from build123d import *

# Parameters (mm, degrees)
BOSS_EXTRUDE1_DEPTH = 3
SKETCH3_R           = 1.55
CUT_EXTRUDE2_DEPTH  = 3
SKETCH4_R           = 1.55
CUT_EXTRUDE4_DEPTH  = 3
SKETCH5_R           = 1.55
CUT_EXTRUDE6_DEPTH  = 3
CUT_EXTRUDE7_DEPTH  = 3


with BuildPart() as part:
    # Sketch1 → Boss-Extrude1 (new body)
    with BuildSketch(Plane.XY):
        with BuildLine():
            Line((-58.058617241, 24.191090517), (41.941382759, 24.191090517))
            ThreePointArc((41.941382759, 24.191090517), (51.941382759, 14.191090517), (41.941382759, 4.191090517))
            Line((41.941382759, 4.191090517), (-58.058617241, 4.191090517))
            ThreePointArc((-58.058617241, 4.191090517), (-68.058617241, 14.191090517), (-58.058617241, 24.191090517))
        make_face()
    extrude(amount=BOSS_EXTRUDE1_DEPTH)

    # Sketch3 → Cut-Extrude2 (cut)
    with BuildSketch(Plane.XY.offset(3)):
        with Locations((-58.058617241, 14.191090517)):
            Circle(SKETCH3_R)
    extrude(amount=-CUT_EXTRUDE2_DEPTH, mode=Mode.SUBTRACT)

    # Sketch4 → Cut-Extrude4 (cut)
    with BuildSketch(Plane(origin=(9.979459273, 1.433252018, 3), x_dir=(1, 0, 0), z_dir=(0, 0, 1))):
        with Locations((-4.038076514, 12.757838499)):
            Circle(SKETCH4_R)
    extrude(amount=-CUT_EXTRUDE4_DEPTH, mode=Mode.SUBTRACT)

    # Sketch5 → Cut-Extrude6 (cut)
    with BuildSketch(Plane(origin=(-9.979459273, 1.433252018, 0), x_dir=(-1, 0, 0), z_dir=(0, 0, -1))):
        with Locations((12.079157968, 12.757838499)):
            Circle(SKETCH5_R)
    extrude(amount=-CUT_EXTRUDE6_DEPTH, mode=Mode.SUBTRACT)

    # Sketch6 → Cut-Extrude7 (cut)
    with BuildSketch(Plane.XY.offset(3)):
        with BuildLine():
            Line((12.606210345, 17.775453704), (41.354831035, 20.463726093))
            ThreePointArc((41.354831035, 20.463726093), (48.241382759, 14.191090517), (41.354831035, 7.918454941))
            Line((41.354831035, 7.918454941), (12.606210345, 10.60672733))
            ThreePointArc((12.606210345, 10.60672733), (9.341382759, 14.191090517), (12.606210345, 17.775453704))
        make_face()
    extrude(amount=-CUT_EXTRUDE7_DEPTH, mode=Mode.SUBTRACT)


solid = part.part
Geometry: final body of the model. Coordinates: model frame, mm. A direction names the side the tool comes from. Give positions to 0.01 mm unless a question says otherwise; leave off trailing zeros. Loops run counter-clockwise (first coordinate to the right, second up) from the corner with the lowest first, then second, coordinate; pieces in that order, holes last. Notation, with made-up numbers: (72.25, 27.5) -> (96.25, 27.5) arc R22 ccw to (96.25, 38.5) -> close; hole circle Ø9 at (29.5, 13.25). An arc over 180 degrees is marked (long way). Put each result on its own line as item: value.
1. Pin query (flat end, axial travel): P1, Ø8, axis at x = -55.5, y = 21.5, coming from the -Z side; P2, Ø11.5, axis at x = 41.94, y = 14.19, coming from the +Z side. Return the tip coordinate at first contact, or that it passes through.
Taken from the geometry:
P1: stops at z = 0
P2: passes through
2. Cut plane B-B (y = 5.5). Return the cut outline in (x, z), plus the area to 3 significant figures.
Taken from the geometry:
outline: (-63, 0) -> (46.89, 0) -> (46.89, 3) -> (-63, 3) -> close
area: 330 mm2
3. Ray query, line 1 along Y through (x, z) = (42.5, 0.55); line 2 along X through (y, z) = (16.25, 1.05); line 3 along X through (y, z) = (14.75, 2.85). Return the intervals inside material, ascending. Write a range as [from, to].
Taken from the geometry:
line 1: y = [4.21, 7.92], [20.47, 24.18]
line 2: x = [-67.84, 9.99], [47.9, 51.73]
line 3: x = [-68.04, -59.5], [-56.61, -23.5], [-20.61, 4.5], [7.39, 9.39], [48.22, 51.93]
4. Pull-direction query (Y, two-part tool) for faces 1 (the flat face through (-7, 4.191, 1)), 2 (the cylindrical face through (48.24, 14.34, 1.52)), 3 (the cylindrical face through (-68.056, 13.971, 1.479)), 4 (the flat face through (-9, 24.191, 1)); classes: released by +Y, released by -Y, zero draft, split by the parting line, or undercut.
Taken from the geometry:
face 1: released by -Y
face 2: undercut
face 3: split by the parting line
face 4: released by +Y
5. Cut plane C-C (y = 22). Return the cut outline in (x, z), plus the area to 3 significant figures.
Taken from the geometry:
outline: (-64.31, 0) -> (48.19, 0) -> (48.19, 3) -> (-64.31, 3) -> close
area: 337 mm2
6. Cut plane A-A (z = 2.05). Return the cut outline in (x, y), plus the area to 3 significant figures.
Taken from the geometry:
outline: (-58.06, 4.19) -> (41.94, 4.19) arc R10 ccw to (41.94, 24.19) -> (-58.06, 24.19) arc R10 ccw to start; hole circle Ø3.1 at (-58.06, 14.19); hole circle Ø3.1 at (-22.06, 14.19); hole circle Ø3.1 at (5.94, 14.19); hole (12.61, 10.61) -> (41.35, 7.92) arc R6.3 ccw (long way) to (41.35, 20.46) -> (12.61, 17.78) arc R3.6 ccw to start
area: 1,920 mm2
7. Set-up query: faces 5 (the flat face through (27.182, 9.244, 1.521)), 6 (the flat face through (-21, 12, 0)). Return all of +Z, -Z, +X, -X, +Y, -Y with unobstructed straight access to the full face (end or side cutting, diameter ignored); none if empty.
Taken from the geometry:
face 5: +Z, -Z
face 6: -Z, +X, -X, +Y, -Y
